Verification items for the finished model (mm, model axes). A direction names the side the tool comes from. Give positions to 0.01 mm unless a question says otherwise; leave off trailing zeros. Write each loop counter-clockwise with the first axis right and the second up, starting at its lowest first coordinate (ties: lowest second). Pieces come first, ordered by that corner, then holes.
from build123d import *

# Parameters (mm, degrees)
SKETCH1_R           = 5
SKETCH1_R_2         = 3
BOSS_EXTRUDE1_DEPTH = 9
CUT_EXTRUDE1_DEPTH  = 9


with BuildPart() as part:
    # Sketch1 → Boss-Extrude1 (new body)
    with BuildSketch(Plane.XY):
        Circle(SKETCH1_R)
        Circle(SKETCH1_R_2, mode=Mode.SUBTRACT)
    extrude(amount=BOSS_EXTRUDE1_DEPTH)

    # Sketch2 → Cut-Extrude1 (cut)
    with BuildSketch(Plane(origin=(0, 0, 0), x_dir=(1, 0, 0), z_dir=(0, 1, 0))):
        Polygon((-5, -3), (0, -3), (0, -6), (3.187015058, -6), (6.391445499, -6), (6.391445499, -9.698491775), (-6.043137843, -9.698491775), (-6.043137843, -2.314369455), (-5, -2.436277134), align=None)
    extrude(amount=CUT_EXTRUDE1_DEPTH, mode=Mode.SUBTRACT)


solid = part.part
Item 1: Depth check by flat-ended pin: pin 1 (1.5 mm diameter, centred on x = -1.5, y = 2, fed in from +Z); pin 2 (0.6 mm diameter, centred on x = 4.5, z = 7.5, fed in from +Y); pin 3 (1.5 mm diameter, centred on x = 1.5, y = 3.5, fed in from +Z); pin 4 (5.5 mm diameter, centred on x = 0, y = 0, fed in from -Z) (3 decimals). Enter the tip coordinate at first touch or a pass-through.
Answer key:
pin 1: stops at z = 3
pin 2: stops at y = 0
pin 3: stops at z = 6
pin 4: passes through
Item 2: Sectioned sample at C-C on z = 8.25. Record the cut outline in (x, y), then the cut area to 3 significant figures.
Answer key:
outline: (-5, 0) arc R5 ccw to (5, 0) - (3, 0) arc R3 cw to (-3, 0) - close
area: 25.1 mm2
Item 3: Sectioned sample at B-B on x = 2. Record the cut outline in (y, z), then the cut area to 3 significant figures.
Answer key:
outline: (-4.58, 0) - (-2.24, 0) - (-2.24, 9) - (-4.58, 9) - close; (2.24, 0) - (4.58, 0) - (4.58, 6) - (2.24, 6) - close
area: 35.2 mm2
Item 4: Sectioned sample at D-D on x = -4. Record the cut outline in (y, z).
Answer key:
outline: (-3, 0) - (3, 0) - (3, 3) - (0, 3) - (0, 9) - (-3, 9) - close
Item 5: Set-up check for faces 5 (the face through (-0.1, -3.3, 0)), 6 (the face through (-4, 0, 6)), 7 (the face through (4, 0, 7)): record each of +Z, -Z, +X, -X, +Y, -Y from which the full face is reachable in a straight line by a thin tool's end or side.
Answer key:
face 5: -Z, +X, -X, +Y, -Y
face 6: +Z, -X, +Y
face 7: +Z, +X, -X, +Y
Item 6: Scan lines: line 1 along Y through (x, z) = (0, 2.75); line 2 along Y through (x, z) = (4, 8.75). Record each from-to range of solid material in increasing order.
Answer key:
line 1: y = -5 to -3, 3 to 5
line 2: y = -3 to 0
Item 7: Sectioned sample at A-A on y = 2. Record the cut outline in (x, z).
Answer key:
outline: (-4.58, 0) - (-2.24, 0) - (-2.24, 3) - (-4.58, 3) - close; (2.24, 0) - (4.58, 0) - (4.58, 6) - (2.24, 6) - close
Item 8: Release check for a two-part mould opening along X. For faces 1 (the face through (3, 2, 6)), 2 (the face through (1.384, -2.662, 3.437)), 3 (the face through (2.307, -4.436, 3.437)), 4 (the face through (0, 4, 4)) record: released by +X, released by -X, zero draft, split by the parting line, or undercut.
Answer key:
face 1: zero draft
face 2: undercut
face 3: split by the parting line
face 4: released by -X
